```python
from build123d import *

# Parameters (mm, degrees)
SKETCH1_R                                           = 23.5
BOSS_EXTRUDE1_DEPTH                                 = 9
BOSS_EXTRUDE1_DEPTH_BACK                            = 0.01
CSK_FOR_M6_COUNTERSUNK_FLAT_HEAD_SCREW1_D           = 6.6
CSK_FOR_M6_COUNTERSUNK_FLAT_HEAD_SCREW1_CSINK_D     = 12.6
CSK_FOR_M6_COUNTERSUNK_FLAT_HEAD_SCREW1_CSINK_ANGLE = 90


with BuildPart() as part:
    # Sketch1 → Boss-Extrude1 (new body, two sides)
    with BuildSketch(Plane(origin=(0, 0, 0), x_dir=(0, 0, -1), z_dir=(1, 0, 0))) as boss_extrude1_sk:
        with BuildLine():
            Line((-25, 110), (25, 110))
            Line((25, 110), (25, 54.543560573))
            ThreePointArc((25, 54.543560573), (0, -60), (-25, 54.543560573))
            Line((-25, 54.543560573), (-25, 110))
        make_face()
        Circle(SKETCH1_R, mode=Mode.SUBTRACT)
    extrude(amount=BOSS_EXTRUDE1_DEPTH)
    extrude(boss_extrude1_sk.sketch, amount=-BOSS_EXTRUDE1_DEPTH_BACK)

    # CSK for M6 Countersunk Flat Head Screw1 (through all)
    with Locations(Plane(origin=(9, 0, 0), x_dir=(0, 0, -1), z_dir=(1, 0, 0))):
        with Locations((-37.476659403, 37.476659403), (0, 53), (37.476659403, 37.476659403), (53, 0), (37.476659403, -37.476659403), (0, -53), (-37.476659403, -37.476659403), (-53, 0)):
            CounterSinkHole(CSK_FOR_M6_COUNTERSUNK_FLAT_HEAD_SCREW1_D / 2, CSK_FOR_M6_COUNTERSUNK_FLAT_HEAD_SCREW1_CSINK_D / 2, counter_sink_angle=CSK_FOR_M6_COUNTERSUNK_FLAT_HEAD_SCREW1_CSINK_ANGLE)


solid = part.part
```
The model under review builds one solid part; all positions refer to its coordinate system, in mm. A direction names the side the tool comes from. Round coordinates to 2 decimals unless told otherwise and drop trailing zeros. Order: outer loops, then holes, each group sorted by start corner. A loop starts at its lowest first (then second) coordinate and runs counter-clockwise, first axis right, second up. Notation, with made-up numbers: (-29.5, 49.5) -> (-12.5, 49.5) arc R7 cw to (-12.5, 59.5) -> close; hole circle Ø2 at (40, 50). An arc over 180 degrees is marked (long way). Use a Markdown table: item, result.
Q1. We need section A-A on y = 0. Write out the cut boundary in (x, z).
Values:
| item | result |
|---|---|
| outline | (-0.01, -60) -> (9, -60) -> (9, -59.3) -> (6, -56.3) -> (-0.01, -56.3) -> close; (-0.01, -49.7) -> (6, -49.7) -> (9, -46.7) -> (9, -23.5) -> (-0.01, -23.5) -> close; (-0.01, 23.5) -> (9, 23.5) -> (9, 46.7) -> (6, 49.7) -> (-0.01, 49.7) -> close; (-0.01, 56.3) -> (6, 56.3) -> (9, 59.3) -> (9, 60) -> (-0.01, 60) -> close |
Q2. Clearance check with flat-ended pins moving along their axes: P1, Ø2.5, axis at x = 5.5, y = 84, coming from the -Z side; P2, Ø8.5, axis at y = -37.48, z = 37.48, coming from the -X side; P3, Ø5, axis at x = 4, y = 63, coming from the +Z side; P4, Ø4, axis at x = 2, y = -10, coming from the +Z side. State where each tip first meets the part, or that it passes through.
Values:
| item | result |
|---|---|
| P1 | stops at z = -25 |
| P2 | stops at x = -0.01 |
| P3 | stops at z = 25 |
| P4 | stops at z = 59.46 |
Q3. Tool access review of faces 1 (the flat face through (5, 83, -25)), 2 (the conical face through (6.146, 38.512, 40.763)), 3 (the flat face through (5, 82, 25)): name each direction out of +Z, -Z, +X, -X, +Y, -Y from which nothing blocks a thin tool from reaching the whole face with its end or side.
Values:
| item | result |
|---|---|
| face 1 | -Z, +X, -X, +Y |
| face 2 | +X |
| face 3 | +Z, +X, -X, +Y |
Q4. We need section B-B on z = 0. Write out the cut boundary in (x, y).
Values:
| item | result |
|---|---|
| outline | (-0.01, -60) -> (9, -60) -> (9, -59.3) -> (6, -56.3) -> (-0.01, -56.3) -> close; (-0.01, -49.7) -> (6, -49.7) -> (9, -46.7) -> (9, -23.5) -> (-0.01, -23.5) -> close; (-0.01, 23.5) -> (9, 23.5) -> (9, 46.7) -> (6, 49.7) -> (-0.01, 49.7) -> close; (-0.01, 56.3) -> (6, 56.3) -> (9, 59.3) -> (9, 110) -> (-0.01, 110) -> close |
Q5. We need section C-C on z = -20. Write out the cut boundary in (x, y).
Values:
| item | result |
|---|---|
| outline | (-0.01, -56.57) -> (9, -56.57) -> (9, -12.34) -> (-0.01, -12.34) -> close; (-0.01, 12.34) -> (9, 12.34) -> (9, 110) -> (-0.01, 110) -> close |
Q6. We need section D-D on x = 2. State how many separate pieces and enclosed holes the cut face has, then the cut area to 3 significant figures.
Values:
| item | result |
|---|---|
| separate pieces | 1 |
| enclosed holes | 9 |
| area | 11,900 mm^2 |
Q7. For line 1 (Y direction, x = 4, z = 0); line 2 (Y direction, x = 8.25, z = 3.5); line 3 (Z direction, x = 2, y = 85), list the stretches that pass through material, from the lowest coordinate up.
Values:
| item | result |
|---|---|
| line 1 | y = -60 to -56.3, -49.7 to -23.5, 23.5 to 49.7, 56.3 to 110 |
| line 2 | y = -59.9 to -57.31, -48.69 to -23.24, 23.24 to 48.69, 57.31 to 110 |
| line 3 | z = -25 to 25 |
Q8. Mouldability with a two-part tool opening along X and no side actions: class faces 4 (the cylindrical face through (2.95, 34.55, -35.95)), 5 (the conical face through (6.146, -35.148, -40.016)) as +X half, -X half, draft (parallel to the pull), parting line (faces both ways), or undercut.
Values:
| item | result |
|---|---|
| face 4 | draft |
| face 5 | +X half |
